Source: CAD feature listing. Evaluate the final solid. Frame: model axes, mm. Face numbers are marked on the shaded views. A direction names the side the tool comes from. Round coordinates to 2 decimals unless told otherwise and drop trailing zeros. Order: outer loops, then holes, each group sorted by start corner. A loop starts at its lowest first (then second) coordinate and runs counter-clockwise, first axis right, second up. Notation, with made-up numbers: M 10,30.25 L 35,30.25 A16 ccw 35,43.25 Z; hole C 58.25,-25.5 d3. An arc over 180 degrees is marked long. Use one line per item in the form item = value. Start each with the question number.
Q1. Section A-A (y = 11.5). Return the cut outline in (x, z), plus the area to 3 significant figures.
Q2. Material intervals for probe 1 along X at (y, z) = (9, 5.5); probe 2 along Z at (x, y) = (11, 8.5); probe 3 along Y at (x, z) = (4.25, 3), sorted ascending.
Q3. Section B-B (z = 5). Return the cut outline in (x, y).
Q4. Section C-C (x = 4.5). Return the cut outline in (y, z), plus the area to 3 significant figures.
Q5. Contact query for flat-ended pins moving along their axis: pin 1 (2 mm diameter, centred on x = 11, z = 2, fed in from +Y); pin 2 (2 mm diameter, centred on x = 11, z = 7, fed in from +Y); pin 3 (3 mm diameter, centred on x = 6.5, y = 12, fed in from +Z). Output: stop coordinate, or through.
Q6. Reachability of the marked faces 1 and 2 from +Z, -Z, +X, -X, +Y, -Y: full face, straight path, thin tool, end or side. Return the list, or none.
Q7. Section D-D (y = 4). Return the cut outline in (x, z), plus the area to 3 significant figures.
Q8. Pull-direction query (X, two-part tool) for the marked faces 3, 4 and 5; classes: pulls with the +X half, pulls with the -X half, needs draft (parallel to the pull), parting line crosses it, or undercut.
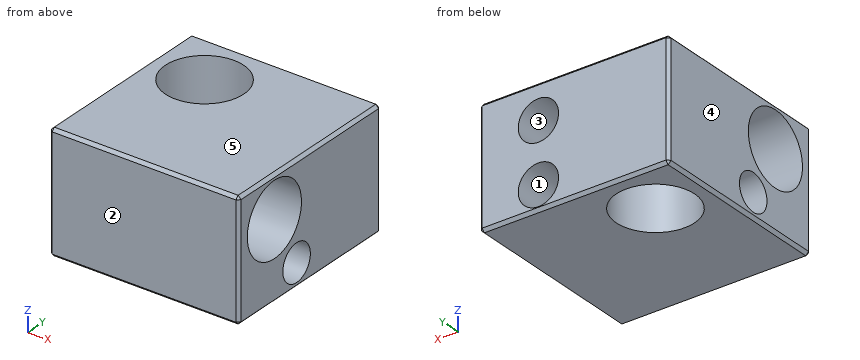
from build123d import *

# Parameters (mm, degrees)
ESQUISSE1_W                     = 16
ESQUISSE1_H                     = 16
BOSS_EXTRU_1_DEPTH              = 10
D_GAGEMENT_M61_D                = 6.6
DIAM_TRE_DU_PER_AGE_6_1_6_1_1_D = 6.1
DIAM_TRE_DU_PER_AGE_3_1_3_1_1_D = 3.1
D_GAGEMENT_M31_D                = 3.4
D_GAGEMENT_M31_DEPTH            = 11
D_GAGEMENT_M31_TIP              = 1.021463052
D_GAGEMENT_M33_D                = 3.4
D_GAGEMENT_M33_DEPTH            = 9.5
D_GAGEMENT_M33_TIP              = 1.021463052
CHANFREIN1_SIZE                 = 0.25


with BuildPart() as part:
    # Esquisse1 → Boss.-Extru.1 (new body)
    with BuildSketch(Plane.XY):
        with Locations((8, 8)):
            Rectangle(ESQUISSE1_W, ESQUISSE1_H)
    extrude(amount=BOSS_EXTRU_1_DEPTH)

    # Dégagement M61 (through all)
    with Locations(Plane.XY.offset(10)):
        with Locations((4.5, 11.5)):
            Hole(D_GAGEMENT_M61_D / 2)

    # Diamètre du perçage Ø6.1 (6.1)1 (through all)
    with Locations(Plane(origin=(16, 0, 0), x_dir=(0, 0, -1), z_dir=(1, 0, 0))):
        with Locations((-6.5, 4)):
            Hole(DIAM_TRE_DU_PER_AGE_6_1_6_1_1_D / 2)

    # Diamètre du perçage Ø3.1 (3.1)1 (through all)
    with Locations(Plane(origin=(16, 0, 0), x_dir=(0, 0, -1), z_dir=(1, 0, 0))):
        with Locations((-2, 6.5)):
            Hole(DIAM_TRE_DU_PER_AGE_3_1_3_1_1_D / 2)

    # Dégagement M31
    with Locations(Plane(origin=(0, 16, 0), x_dir=(1, 0, 0), z_dir=(0, 1, 0))):
        with Locations((11, -7)):
            Hole(D_GAGEMENT_M31_D / 2, depth=D_GAGEMENT_M31_DEPTH)
            with Locations((0, 0, -(D_GAGEMENT_M31_DEPTH + D_GAGEMENT_M31_TIP / 2))):  # 118° drill point
                Cone(0, D_GAGEMENT_M31_D / 2, D_GAGEMENT_M31_TIP, mode=Mode.SUBTRACT)

    # Dégagement M33
    with Locations(Plane(origin=(0, 16, 0), x_dir=(1, 0, 0), z_dir=(0, 1, 0))):
        with Locations((11, -2)):
            Hole(D_GAGEMENT_M33_D / 2, depth=D_GAGEMENT_M33_DEPTH)
            with Locations((0, 0, -(D_GAGEMENT_M33_DEPTH + D_GAGEMENT_M33_TIP / 2))):  # 118° drill point
                Cone(0, D_GAGEMENT_M33_D / 2, D_GAGEMENT_M33_TIP, mode=Mode.SUBTRACT)

    # Chanfrein1
    chanfrein1_edges = [part.edges().sort_by_distance(p)[0] for p in [
        (16, 8, 10),
        (8, 16, 10),
        (0, 8, 10),
        (8, 16, 0),
        (16, 8, 0),
        (8, 0, 0),
        (0, 8, 0),
        (8, 0, 10),
        (0, 16, 5),
        (16, 16, 5),
        (16, 0, 5),
        (0, 0, 5),
    ]]
    chamfer(chanfrein1_edges, length=CHANFREIN1_SIZE)


solid = part.part
Results list:
q1.outline = M 0,0.25 L 0.25,0 L 1.2,0 L 1.2,10 L 0.25,10 L 0,9.75 Z; M 7.8,0 L 15.75,0 L 16,0.25 L 16,9.75 L 15.75,10 L 7.8,10 Z; hole C 11,2 d3.4; hole C 11,7 d3.4
q1.area = 75.7 mm2
q2.probe_1 = 0 to 2.35, 6.65 to 10.2, 11.8 to 16
q2.probe_2 = 0 to 0.3, 3.7 to 5.3, 8.7 to 10
q2.probe_3 = 0 to 5.32, 7.68 to 8.21, 14.79 to 16
q3.outline = M 0,0.25 L 0.25,0 L 15.75,0 L 16,0.25 L 16,1.34 L 0,1.34 Z; M 0,6.66 L 16,6.66 L 16,15.75 L 15.75,16 L 0.25,16 L 0,15.75 Z; hole C 4.5,11.5 d6.6
q4.outline = M 0,0.25 L 0.25,0 L 8.2,0 L 8.2,10 L 0.25,10 L 0,9.75 Z; M 14.8,0 L 15.75,0 L 16,0.25 L 16,9.75 L 15.75,10 L 14.8,10 Z; hole C 4,6.5 d6.1; hole C 6.5,2 d3.1
q4.area = 57.1 mm2
q5.pin_1 = 5.32
q5.pin_2 = 1.34
q5.pin_3 = 10
q6.face_1 = +Y
q6.face_2 = +Z, -Z, +X, -X, -Y
q7.outline = M 0,0.25 L 0.25,0 L 15.75,0 L 16,0.25 L 16,3.45 L 0,3.45 Z; M 0,9.55 L 16,9.55 L 16,9.75 L 15.75,10 L 0.25,10 L 0,9.75 Z
q7.area = 62.3 mm2
q8.face_3 = undercut
q8.face_4 = pulls with the -X half
q8.face_5 = needs draft
